Check sheet for the modelled part. Datum: model origin and axes. Units: mm. Round coordinates to 2 decimals unless told otherwise and drop trailing zeros. Write each loop counter-clockwise with the first axis right and the second up, starting at its lowest first coordinate (ties: lowest second). Pieces come first, ordered by that corner, then holes. Notation, with made-up numbers: (-31.75, 16.5) -> (-17.75, 16.5) arc R23 ccw to (-17.75, 38.5) -> close; hole circle Ø8 at (35.5, 18). An arc over 180 degrees is marked (long way). Write item = value, one per line.
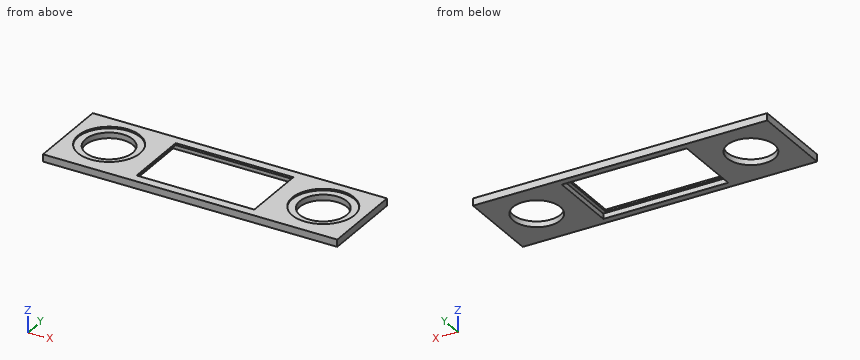
from build123d import *

# Parameters (mm, degrees)
SKETCH2_W           = 735
SKETCH2_H           = 210
SKETCH2_R           = 59
SKETCH2_W_2         = 294
SKETCH2_H_2         = 165
BOSS_EXTRUDE1_DEPTH = 18
SKETCH3_R           = 77.5
CUT_EXTRUDE1_DEPTH  = 4
SKETCH4_W           = 312
SKETCH4_H           = 175
CUT_EXTRUDE2_DEPTH  = 13


with BuildPart() as part:
    # Sketch2 → Boss-Extrude1 (new body)
    with BuildSketch(Plane.XY):
        Rectangle(SKETCH2_W, SKETCH2_H)
        with Locations((-267.5, 5)):
            Circle(SKETCH2_R, mode=Mode.SUBTRACT)
        with Locations((267.5, 5)):
            Circle(SKETCH2_R, mode=Mode.SUBTRACT)
        Rectangle(SKETCH2_W_2, SKETCH2_H_2, mode=Mode.SUBTRACT)
    extrude(amount=BOSS_EXTRUDE1_DEPTH)

    # Sketch3 → Cut-Extrude1 (cut)
    with BuildSketch(Plane.XY.offset(18)):
        with Locations((-267.5, 5)):
            Circle(SKETCH3_R)
        with Locations((267.5, 5)):
            Circle(SKETCH3_R)
    extrude(amount=-CUT_EXTRUDE1_DEPTH, mode=Mode.SUBTRACT)

    # Sketch4 → Cut-Extrude2 (cut)
    with BuildSketch(Plane(origin=(0, 0, 0), x_dir=(-1, 0, 0), z_dir=(0, 0, -1))):
        Rectangle(SKETCH4_W, SKETCH4_H)
    extrude(amount=-CUT_EXTRUDE2_DEPTH, mode=Mode.SUBTRACT)


solid = part.part
(1) Material ranges on L1, parallel to X at y = 5, z = 8.75; L2, parallel to X at y = 42, z = 14.5; L3, parallel to Y at x = 267.5, z = 8, recorded low to high. Write a range as [from, to].
Worked answers:
L1 = [-367.5, -326.5], [-208.5, -156], [156, 208.5], [326.5, 367.5]
L2 = [-367.5, -335.6], [-199.4, -147], [147, 199.4], [335.6, 367.5]
L3 = [-105, -54], [64, 105]
(2) Sectioned sample at D-D on x = 267.5. Enter the section's corners in (y, z), then the cut area to 3 significant figures.
Worked answers:
outline = (-105, 0) -> (-54, 0) -> (-54, 14) -> (-72.5, 14) -> (-72.5, 18) -> (-105, 18) -> close; (64, 0) -> (105, 0) -> (105, 18) -> (82.5, 18) -> (82.5, 14) -> (64, 14) -> close
area = 1,510 mm²
(3) Sectioned sample at C-C on y = 5. Enter the section's corners in (x, z).
Worked answers:
outline = (-367.5, 0) -> (-326.5, 0) -> (-326.5, 14) -> (-345, 14) -> (-345, 18) -> (-367.5, 18) -> close; (-208.5, 0) -> (-156, 0) -> (-156, 13) -> (-147, 13) -> (-147, 18) -> (-190, 18) -> (-190, 14) -> (-208.5, 14) -> close; (147, 13) -> (156, 13) -> (156, 0) -> (208.5, 0) -> (208.5, 14) -> (190, 14) -> (190, 18) -> (147, 18) -> close; (326.5, 0) -> (367.5, 0) -> (367.5, 18) -> (345, 18) -> (345, 14) -> (326.5, 14) -> close
(4) Sectioned sample at B-B on z = 7.5. Enter the section's corners in (x, y).
Worked answers:
outline = (-367.5, -105) -> (367.5, -105) -> (367.5, 105) -> (-367.5, 105) -> close; hole circle Ø118 at (-267.5, 5); hole (-156, -87.5) -> (156, -87.5) -> (156, 87.5) -> (-156, 87.5) -> close; hole circle Ø118 at (267.5, 5)
(5) Go/stop test with a flat-tipped pin: P1, Ø3, axis at x = -217, y = 62, coming from the +Z side. Record where the tip stops, or that it passes through.
Worked answers:
P1 = 18
(6) Sectioned sample at A-A on x = 128.5. Enter the section's corners in (y, z).
Worked answers:
outline = (-105, 0) -> (-87.5, 0) -> (-87.5, 13) -> (-82.5, 13) -> (-82.5, 18) -> (-105, 18) -> close; (82.5, 13) -> (87.5, 13) -> (87.5, 0) -> (105, 0) -> (105, 18) -> (82.5, 18) -> close
